Verification items for this drawing (mm, ordinates from the low corner). Round coordinates to 2 decimals unless told otherwise and drop trailing zeros. Order: outer loops, then holes, each group sorted by start corner. A loop starts at its lowest first (then second) coordinate and runs counter-clockwise, first axis right, second up.
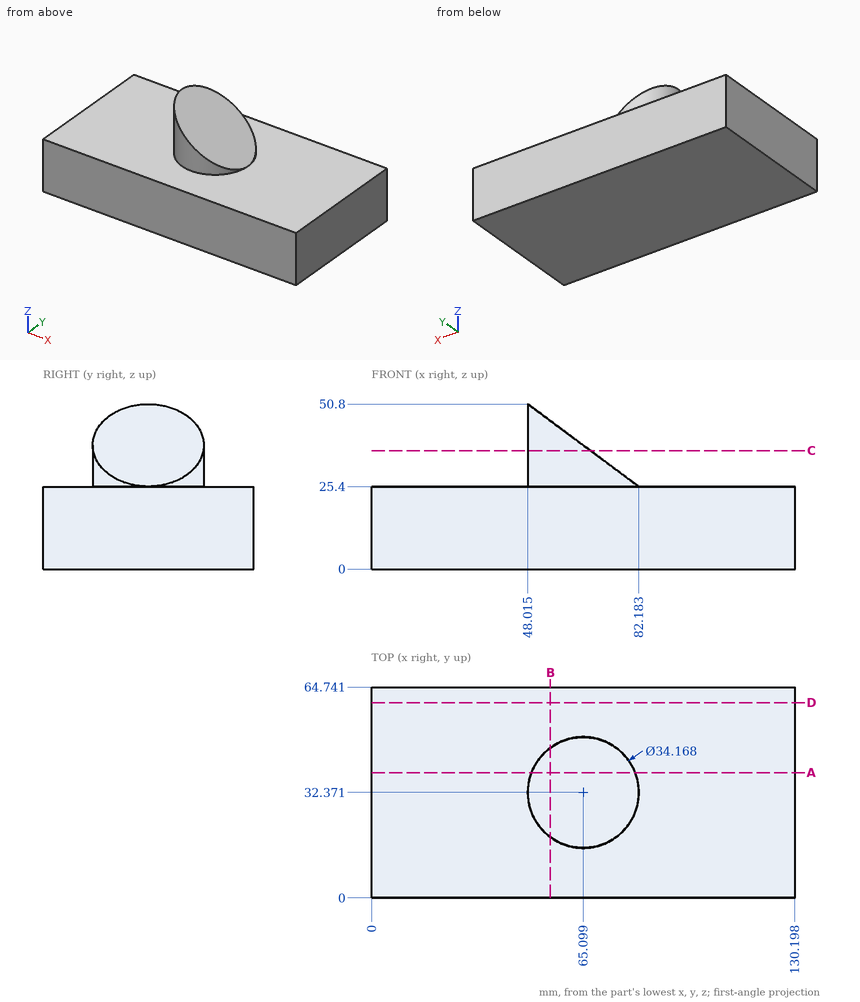
Item 1: Sectioned sample at D-D (y = 60). Record the cut outline in (x, z), and give its area (3 significant figures).
Answer:
outline: (0, 0) - (130.2, 0) - (130.2, 25.4) - (0, 25.4) - close
area: 3,310 mm2
Item 2: Sectioned sample at C-C (z = 36.5). Record the cut outline in (x, y).
Answer:
outline: (67.25, 15.42) - (67.25, 49.32) arc R17.08 ccw (long way) to start
Item 3: Sectioned sample at B-B (x = 55). Record the cut outline in (y, z).
Answer:
outline: (0, 0) - (64.74, 0) - (64.74, 25.4) - (46.15, 25.4) - (46.15, 45.61) - (18.59, 45.61) - (18.59, 25.4) - (0, 25.4) - close
Item 4: Scan lines: line 1 along Z through (x, y) = (52, 54); line 2 along Z through (x, y) = (58.5, 29) (1 decimal); line 3 along X through (y, z) = (38, 30) (1 decimal). Record each from-to range of solid material in increasing order.
Answer:
line 1: z = 0 to 25.4
line 2: z = 0 to 43
line 3: x = 49 to 76
Item 5: Sectioned sample at A-A (y = 38.5). Record the cut outline in (x, z) (1 decimal).
Answer:
outline: (0, 0) - (130.2, 0) - (130.2, 25.4) - (81, 25.4) - (81, 26.2) - (49.2, 50) - (49.2, 25.4) - (0, 25.4) - close
Item 6: Go/stop test with flat-tipped pins: P1, Ø19.5, axis at x = 80.5, y = 35, coming from the +Z side; P2, Ø3, axis at x = 20.5, y = 32, coming from the -Z side; P3, Ø4, axis at y = 33.5, z = 33, coming from the +X side; P4, Ø5, axis at y = 50.5, z = 29, coming from the -X side. Record where each tip stops, or that it passes through.
Answer:
P1: stops at z = 33.9
P2: stops at z = 0
P3: stops at x = 74.65
P4: stops at x = 58.2
